Geometry check sheet. Reference: the model listing, model coordinates, mm. A direction names the side the tool comes from. Coordinates: 2 decimals unless noted, no trailing zeros. Loops run counter-clockwise (first coordinate to the right, second up) from the corner with the lowest first, then second, coordinate; pieces in that order, holes last. Notation, with made-up numbers: (11, -17.5) - (67, -17.5) arc R37 ccw to (67, 21.5) - close; hole circle Ø3 at (56, 30.25). An arc over 180 degrees is marked (long way). Write item = value, one per line. Start each with the question number.
from build123d import *

# Parameters (mm, degrees)
SKETCH_1_W           = 170
SKETCH_1_H           = 100
EXTRUDE_1_DEPTH      = 5
SKETCH_3_R           = 1.5
CUT_EXTRUDE_2_DEPTH  = 99.742088291
SKETCH_5_R           = 22.5
CUT_EXTRUDE_4_DEPTH  = 99.742088291
SKETCH_6_W           = 170
SKETCH_6_H           = 6
CUT_EXTRUDE_5_DEPTH  = 99.742088291
SKETCH_7_R           = 2.5
CUT_EXTRUDE_6_DEPTH  = 99.742088291
SKETCH_8_W           = 170
SKETCH_8_H           = 18
CUT_EXTRUDE_7_DEPTH  = 10
SKETCH_9_W           = 18
SKETCH_9_H           = 12
CUT_EXTRUDE_9_DEPTH  = 10
SKETCH_10_W          = 18
SKETCH_10_H          = 12
CUT_EXTRUDE_10_DEPTH = 10
FILLET_3_R           = 3
SKETCH_11_W          = 170
SKETCH_11_H          = 5
EXTRUDE_2_DEPTH      = 10
FILLET_4_R           = 3
FILLET_5_R           = 10
SKETCH_12_R          = 1.6
CUT_EXTRUDE_11_DEPTH = 96.843622636
SKETCH_13_R          = 2
CUT_EXTRUDE_12_DEPTH = 17


with BuildPart() as part:
    # 草图1 → 凸台-拉伸1 (new body)
    with BuildSketch(Plane.XY):
        Rectangle(SKETCH_1_W, SKETCH_1_H)
    extrude(amount=EXTRUDE_1_DEPTH)

    # 草图3 → 切除-拉伸2 (cut, through all)
    with BuildSketch(Plane.XY.offset(5)):
        with Locations((-77, 22)):
            Circle(SKETCH_3_R)
        with Locations((-77, -22)):
            Circle(SKETCH_3_R)
        with Locations((77, 22)):
            Circle(SKETCH_3_R)
        with Locations((76.972177567, -21.999991204)):
            Circle(SKETCH_3_R)
        with Locations((-77, 15)):
            Circle(SKETCH_3_R)
        with Locations((-77, 5)):
            Circle(SKETCH_3_R)
        with Locations((-76.95458974, -4.999896895)):
            Circle(SKETCH_3_R)
        with Locations((-76.973665901, -14.9998787)):
            Circle(SKETCH_3_R)
        with Locations((77, 14.9999673)):
            Circle(SKETCH_3_R)
        with Locations((76.999998846, 4.9999673)):
            Circle(SKETCH_3_R)
        with Locations((77.000079735, -5.000032699)):
            Circle(SKETCH_3_R)
        with Locations((76.996042364, -15.000031884)):
            Circle(SKETCH_3_R)
    extrude(amount=-CUT_EXTRUDE_2_DEPTH, mode=Mode.SUBTRACT)

    # 草图5 → 切除-拉伸4 (cut, through all)
    with BuildSketch(Plane.XY.offset(5)):
        with Locations((0, -5)):
            Circle(SKETCH_5_R)
    extrude(amount=-CUT_EXTRUDE_4_DEPTH, mode=Mode.SUBTRACT)

    # 草图6 → 切除-拉伸5 (cut, through all)
    with BuildSketch(Plane.XY.offset(5)):
        with Locations((0, -47)):
            Rectangle(SKETCH_6_W, SKETCH_6_H)
    extrude(amount=-CUT_EXTRUDE_5_DEPTH, mode=Mode.SUBTRACT)

    # 草图7 → 切除-拉伸6 (cut, through all)
    with BuildSketch(Plane.XY.offset(5)):
        with Locations((30, -32)):
            Circle(SKETCH_7_R)
        with Locations((-30, -32)):
            Circle(SKETCH_7_R)
    extrude(amount=-CUT_EXTRUDE_6_DEPTH, mode=Mode.SUBTRACT)

    # 草图8 → 切除-拉伸7 (cut)
    with BuildSketch(Plane.XY.offset(5)):
        with Locations((0, 41)):
            Rectangle(SKETCH_8_W, SKETCH_8_H)
    extrude(amount=-CUT_EXTRUDE_7_DEPTH, mode=Mode.SUBTRACT)

    # 草图9 → 切除-拉伸9 (cut)
    with BuildSketch(Plane.XY.offset(5)):
        with Locations((-63, 26)):
            Rectangle(SKETCH_9_W, SKETCH_9_H)
        with Locations((63, 26)):
            Rectangle(SKETCH_9_W, SKETCH_9_H)
    extrude(amount=-CUT_EXTRUDE_9_DEPTH, mode=Mode.SUBTRACT)

    # 草图10 → 切除-拉伸10 (cut)
    with BuildSketch(Plane.XY.offset(5)):
        with Locations((-63, -26)):
            Rectangle(SKETCH_10_W, SKETCH_10_H)
        with Locations((63, -26)):
            Rectangle(SKETCH_10_W, SKETCH_10_H)
    extrude(amount=-CUT_EXTRUDE_10_DEPTH, mode=Mode.SUBTRACT)

    # 圆角3
    fillet_3_edges = [part.edges().sort_by_distance(p)[0] for p in [
        (-54, 20, 2.5),
        (-72, 20, 2.5),
        (54, 20, 2.5),
        (72, 20, 2.5),
        (-72, -32, 2.5),
        (-72, -20, 2.5),
        (-54, -20, 2.5),
        (-54, -32, 2.5),
        (72, -20, 2.5),
        (72, -32, 2.5),
        (54, -32, 2.5),
        (54, -20, 2.5),
    ]]
    fillet(fillet_3_edges, radius=FILLET_3_R)

    # 草图11 → 凸台-拉伸2 (add)
    with BuildSketch(Plane(origin=(0, 32, 0), x_dir=(1, 0, 0), z_dir=(0, 1, 0))):
        with Locations((0, -2.5)):
            Rectangle(SKETCH_11_W, SKETCH_11_H)
    extrude(amount=EXTRUDE_2_DEPTH)

    # 圆角4
    fillet_4_edges = [part.edges().sort_by_distance(p)[0] for p in [
        (-72, 32, 2.5),
        (-54, 32, 2.5),
        (54, 32, 2.5),
        (72, 32, 2.5),
    ]]
    fillet(fillet_4_edges, radius=FILLET_4_R)

    # 圆角5
    fillet_5_edges = [part.edges().sort_by_distance(p)[0] for p in [
        (-85, 42, 2.5),
        (85, 42, 2.5),
        (-85, -44, 2.5),
        (85, -44, 2.5),
    ]]
    fillet(fillet_5_edges, radius=FILLET_5_R)

    # 草图12 → 切除-拉伸11 (cut, through all)
    with BuildSketch(Plane.XY.offset(5)):
        with Locations((-49, 22)):
            Circle(SKETCH_12_R)
        with Locations((-49, 15)):
            Circle(SKETCH_12_R)
        with Locations((-48.973665901, -15)):
            Circle(SKETCH_12_R)
        with Locations((-49, -22)):
            Circle(SKETCH_12_R)
        with Locations((49, 22)):
            Circle(SKETCH_12_R)
        with Locations((49, 15)):
            Circle(SKETCH_12_R)
        with Locations((48.973665901, -15)):
            Circle(SKETCH_12_R)
        with Locations((49, -22)):
            Circle(SKETCH_12_R)
    extrude(amount=-CUT_EXTRUDE_11_DEPTH, mode=Mode.SUBTRACT)

    # 草图13 → 切除-拉伸12 (cut)
    with BuildSketch(Plane.XY.offset(5)):
        with Locations((25.980762114, 10)):
            Circle(SKETCH_13_R)
        with Locations((25.980762114, -20)):
            Circle(SKETCH_13_R)
        with Locations((0, 25)):
            Circle(SKETCH_13_R)
        with Locations((0, -35)):
            Circle(SKETCH_13_R)
        with Locations((-25.980762114, 10)):
            Circle(SKETCH_13_R)
        with Locations((-25.980762114, -20)):
            Circle(SKETCH_13_R)
    extrude(amount=-CUT_EXTRUDE_12_DEPTH, mode=Mode.SUBTRACT)


solid = part.part
(1) Sectioned sample at C-C on z = 2.9. Count the separate pieces of the cut face and the enclosed holes in it, plus the area to 3 significant figures.
(2) Sectioned sample at A-A on x = 62. Enter the section's corners in (y, z).
(3) Scan lines: line 1 (Y direction, x = 26, z = 3.4); line 2 (X direction, y = 28.5, z = 3.35); line 3 (Y direction, x = 49.5, z = 1.2). Record each from-to range of solid material in increasing order.
(4) Sectioned sample at B-B on x = 30. Enter the section's corners in (y, z), plus the area to 3 significant figures.
(5) Draft check along X on faces 3 (the face through (78.386, 14.425, 2.535)), 4 (the face through (-1, 18, 5)), 5 (the face through (85, -1, 3)). Enter one of: pulls with the +X half, pulls with the -X half, needs draft (parallel to the pull), parting line crosses it, or undercut.
(6) Tool access check on faces 1 (the face through (-71.1, -20.86, 2.46)), 2 (the face through (-81.99, -41.15, 2.46)). Record the directions out of +Z, -Z, +X, -X, +Y, -Y that give a thin tool (end or side, any length) a straight path to the whole face; none if there is none.
Working result:
q1.separate_pieces = 1
q1.enclosed_holes = 33
q1.area = 11,800 mm2
q2.outline = (-44, 0) - (-32, 0) - (-32, 5) - (-44, 5) - close; (-20, 0) - (20, 0) - (20, 5) - (-20, 5) - close; (32, 0) - (42, 0) - (42, 5) - (32, 5) - close
q3.line_1 = -44 to -22, -18 to 8, 12 to 42
q3.line_2 = -85 to -72, -54 to 54, 72 to 85
q3.line_3 = -44 to -23.52, -20.48 to -16.51, -13.49 to 13.48, 16.52 to 20.48, 23.52 to 42
q4.outline = (-44, 0) - (-34.5, 0) - (-34.5, 5) - (-44, 5) - close; (-29.5, 0) - (42, 0) - (42, 5) - (-29.5, 5) - close
q4.area = 405 mm2
q5.face_3 = undercut
q5.face_4 = needs draft
q5.face_5 = pulls with the +X half
q6.face_1 = +Z, -Z
q6.face_2 = +Z, -Z, -X, -Y
